Read the model definition and answer for the solid it produces. Units are mm, in the model's axes. A direction names the side the tool comes from. Coordinates: 2 decimals unless noted, no trailing zeros. Order: outer loops, then holes, each group sorted by start corner. A loop starts at its lowest first (then second) coordinate and runs counter-clockwise, first axis right, second up. Notation, with made-up numbers: M -6,-17 L 8,-17 A10 cw 8,2 Z; hole C 13.25,16 d4. An arc over 180 degrees is marked long. One line per question, with ' | ' between items. Start each with the question number.
1) Find section A-A, the plane z = 0. Write down the section's boundary in (x, y).
2) Find section B-B, the plane x = 0. Write down the section's boundary in (y, z).
3) A tool of negligible diameter and unlimited length cuts with its end or side. For faces 1 (the face through (-3.905, -4.437, -0.867)), 2 (the face through (0, -10, 0)), from which of +Z, -Z, +X, -X, +Y, -Y can it reach the whole face along a straight path? Write none if from no direction.
4) Find section C-C, the plane y = -4.25. Write down the section's boundary in (x, z).
5) Consider probe 1 along X at (y, z) = (0.5, 3); probe 2 along X at (y, z) = (-5.25, 1.25); probe 3 along Z at (x, y) = (-1.75, -2). Determine where each line is inside the solid, lowest interval first.
6) Given P1, Ø1.5, axis at x = 1, y = -0.5, coming from the -Z side; P2, Ø6, axis at x = 0.5, y = -7, coming from the -Z side; P3, Ø3, axis at y = -3, z = 1, coming from the +X side, each flat-ended and moving along its own axis, determine where each tip first touches the part or whether it passes through.
7) Find section D-D, the plane y = 0.5. Write down the section's boundary in (x, z), plus the area to 3 significant figures.
from build123d import *

# Parameters (mm, degrees)
ESBO_O1_R       = 4
EXTRUS_O1_DEPTH = 10
ESBO_O2_R       = 5
EXTRUS_O2_DEPTH = 2
CHANFRO1_SIZE   = 1
CHANFRO2_SIZE   = 1


with BuildPart() as part:
    # Esboço1 → Extrusão1 (new body)
    with BuildSketch(Plane(origin=(0, 0, 0), x_dir=(1, 0, 0), z_dir=(0, 1, 0))):
        with Locations(Location((0, 0, 0), (0, 0, 270))):  # turned: the seam where the file's is
            Circle(ESBO_O1_R)
    extrude(amount=-EXTRUS_O1_DEPTH)

    # Esboço2 → Extrusão2 (add)
    with BuildSketch(Plane(origin=(0, 0, 0), x_dir=(1, 0, 0), z_dir=(0, 1, 0))):
        with Locations(Location((0, 0, 0), (0, 0, 270))):  # turned: the seam where the file's is
            Circle(ESBO_O2_R)
    extrude(amount=EXTRUS_O2_DEPTH)

    # Chanfro1
    chanfro1_edges = [part.edges().sort_by_distance(p)[0] for p in [
        (0, -10, -4),
    ]]
    chamfer(chanfro1_edges, length=CHANFRO1_SIZE)

    # Chanfro2
    chanfro2_edges = [part.edges().sort_by_distance(p)[0] for p in [
        (0, 2, -5),
    ]]
    chamfer(chanfro2_edges, length=CHANFRO2_SIZE)


solid = part.part
Report:
1) outline: M -5,0 L -4,0 L -4,-9 L -3,-10 L 3,-10 L 4,-9 L 4,0 L 5,0 L 5,1 L 4,2 L -4,2 L -5,1 Z
2) outline: M -10,-3 L -9,-4 L 0,-4 L 0,-5 L 1,-5 L 2,-4 L 2,4 L 1,5 L 0,5 L 0,4 L -9,4 L -10,3 Z
3) face 1: -Y | face 2: +Z, -Z, +X, -X, -Y
4) outline: C 0,0 d8
5) probe 1: x = -4 to 4 | probe 2: x = -3.8 to 3.8 | probe 3: z = -3.6 to 3.6
6) P1: stops at z = -4.98 | P2: stops at z = -4 | P3: stops at x = 4
7) outline: C 0,0 d10 | area: 78.5 mm^2
